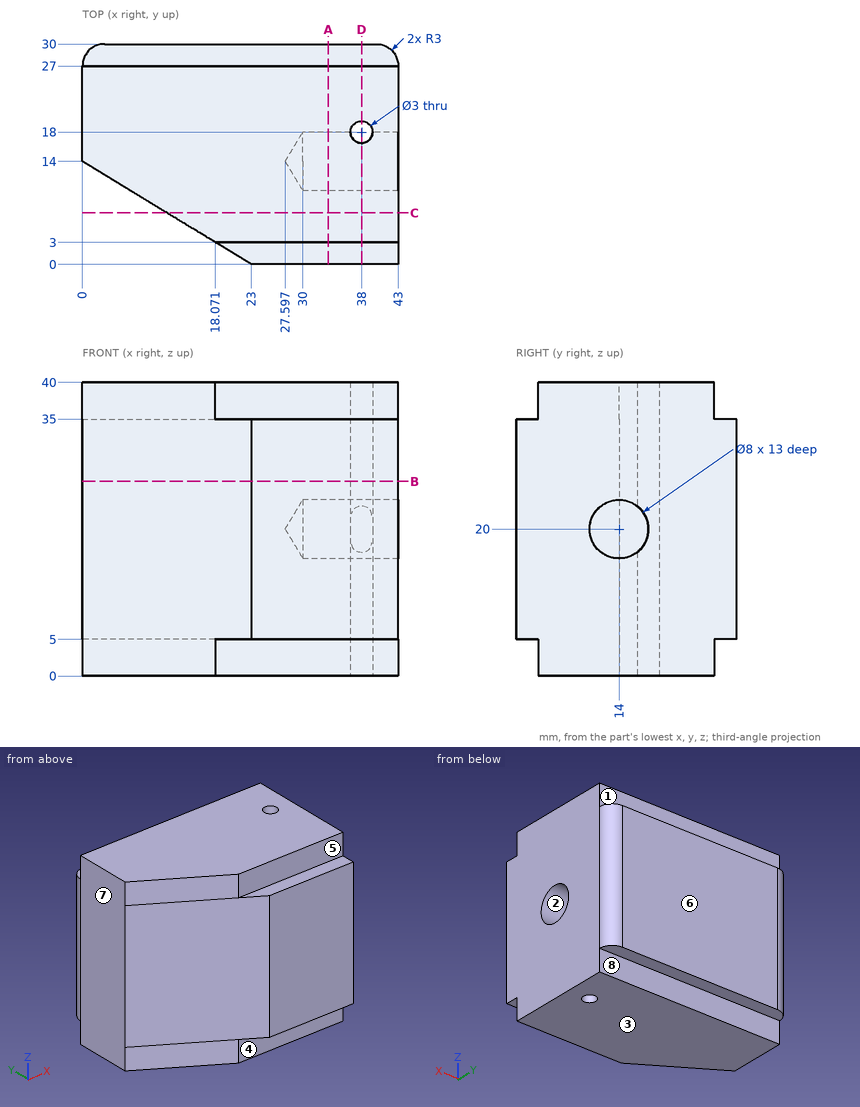
Verification items for this drawing (mm, ordinates from the low corner). A direction names the side the tool comes from. Coordinates: 2 decimals unless noted, no trailing zeros. Loops run counter-clockwise (first coordinate to the right, second up) from the corner with the lowest first, then second, coordinate; pieces in that order, holes last. Notation, with made-up numbers: (-7.75, 1.25) -> (18.25, 1.25) arc R24 ccw to (18.25, 26.25) -> close; hole circle Ø1 at (-31.75, 49.25). An arc over 180 degrees is marked (long way). Put each result on its own line as item: value.
1. Mould release check, pull along Z, two halves, no side actions. Record for the marked faces 1, 2 and 3: pulls with the +Z half, pulls with the -Z half, needs draft (parallel to the pull), parting line crosses it, or undercut.
Result set:
face 1: needs draft
face 2: undercut
face 3: pulls with the -Z half
2. Section check A-A, the plane x = 33.5. Record the boundary of the cut face in (y, z), then the cut area to 3 significant figures.
Result set:
outline: (0, 5) -> (3, 5) -> (3, 0) -> (27, 0) -> (27, 5) -> (30, 5) -> (30, 35) -> (27, 35) -> (27, 40) -> (3, 40) -> (3, 35) -> (0, 35) -> close; hole circle Ø8 at (14, 20)
area: 1,090 mm^2
3. Tool access check on the marked faces 4, 5, 6, 7 and 8. Record the directions out of +Z, -Z, +X, -X, +Y, -Y that give a thin tool (end or side, any length) a straight path to the whole face; none if there is none.
Result set:
face 4: -Z, +X, -X, -Y
face 5: +Z, +X, -X, -Y
face 6: +Z, -Z, +X, -X, +Y
face 7: +Z, -Z, -X, +Y, -Y
face 8: -Z, +X, -X, +Y
4. Section check B-B, the plane z = 26.5. Record the boundary of the cut face in (x, y), then the cut area to 3 significant figures.
Result set:
outline: (0, 14) -> (23, 0) -> (43, 0) -> (43, 27) arc R3 ccw to (40, 30) -> (3, 30) arc R3 ccw to (0, 27) -> close; hole circle Ø3 at (38, 18)
area: 1,120 mm^2
5. Section check C-C, the plane y = 7. Record the boundary of the cut face in (x, z).
Result set:
outline: (11.5, 0) -> (43, 0) -> (43, 40) -> (11.5, 40) -> close
6. Thickness scan on line 1 (Y direction, x = 38, z = 14); line 2 (Y direction, x = 35.25, z = 20); line 3 (X direction, y = 18, z = 15.5). Record the ranges inside material, lowest first.
Result set:
line 1: y = 0 to 16.5, 19.5 to 30
line 2: y = 0 to 10, 18 to 30
line 3: x = 0 to 36.5, 39.5 to 43
7. Section check D-D, the plane x = 38. Record the boundary of the cut face in (y, z).
Result set:
outline: (0, 5) -> (3, 5) -> (3, 0) -> (16.5, 0) -> (16.5, 16.88) arc R4 cw (long way) to (16.5, 23.12) -> (16.5, 40) -> (3, 40) -> (3, 35) -> (0, 35) -> close; (19.5, 0) -> (27, 0) -> (27, 5) -> (30, 5) -> (30, 35) -> (27, 35) -> (27, 40) -> (19.5, 40) -> close
8. Gauge pin test, flat ends, axial feed: P1, Ø1.5, axis at x = 28, y = 1.5, coming from the +Z side; P2, Ø1, axis at y = 12.5, z = 7, coming from the -X side (1 decimal); P3, Ø4, axis at x = 27.5, z = 2.5, coming from the -Y side. Record the tip position at first contact, or that the pin passes through.
Result set:
P1: stops at z = 35
P2: stops at x = 1.6
P3: stops at y = 3
